Input: part model. Units: mm. Frame: model coordinates. A direction names the side the tool comes from. Round coordinates to 2 decimals unless told otherwise and drop trailing zeros. Loops run counter-clockwise (first coordinate to the right, second up) from the corner with the lowest first, then second, coordinate; pieces in that order, holes last. Notation, with made-up numbers: M -17,8.25 L 8,8.25 A25 cw 8,25.25 Z; hole C -30.5,66.5 d11. An arc over 180 degrees is marked long. Use one line per item in the form item = value. Start each with the question number.
Q1. Access query for faces 1 (the flat face through (24, 1, 0)), 2 (the flat face through (-46, 12.7, 82)), 3 (the flat face through (25, 1, 25.4)). Directions: +Z, -Z, +X, -X, +Y, -Y. A direction counts if a zero-diameter tool reaches every point of the face in a straight line with its end or side. Return the directions, or none.
Q2. Section query B-B, the plane z = 75. Output: boundary loops of the cut face in (x, y), and give its area (3 significant figures).
Q3. Section query A-A, the plane x = -0.5. Output: boundary loops of the cut face in (y, z), and give its area (3 significant figures).
Q4. First-contact query: P1, Ø5, axis at y = 14.5, z = 107.5, coming from the +X side; P2, Ø3, axis at x = -18.5, y = 2, coming from the +Z side; P3, Ø4, axis at x = -41.5, y = -29.5, coming from the +Z side. Flat tips, straight axial feed; report the tip coordinate or a pass-through.
Q5. Section query D-D, the plane y = 19.5. Output: boundary loops of the cut face in (x, z).
Q6. Mould query, pull axis X, two halves, no side actions, for faces 4 (the cylindrical face through (-45.87, -43.16, 119.76)), 5 (the cylindrical face through (6.72, 40.54, 12.88)), 6 (the flat face through (-58.395, 23, 83)), 7 (the flat face through (62.344, 44.361, 12.522)). Classes: pulls with the +X half, pulls with the -X half, needs draft (parallel to the pull), parting line crosses it, or undercut.
Q7. Ray query, line 1 along Y through (x, z) = (50, 7); line 2 along Y through (x, z) = (0, 19); line 3 along Z through (x, y) = (42.5, 4). Return the intervals inside material, ascending.
Q8. Section query C-C, the plane y = -30. Output: boundary loops of the cut face in (x, z).
```python
from build123d import *

# Parameters (mm, degrees)
F1_DEPTH      = 50.8
F1_DEPTH_BACK = 50.8
F3_DEPTH      = 25.4
F4_R          = 12.5
F5_DEPTH      = 25.4
F6_R          = 25.4
F7_SIZE       = 12.7


with BuildPart() as f1:
    # F0 (on Front) → F1 (new body, two sides)
    with BuildSketch(Plane.XZ) as f1_sk:
        with BuildLine():
            Line((-32.9945316374, 127), (-58.3945316374, 127))
            Line((-58.3945316374, 127), (-58.3945316374, 38.1))
            ThreePointArc((-58.3945316374, 38.1), (-47.2353000006, 11.1592316368), (-20.2945316374, 0))
            Line((-20.2945316374, 0), (68.6054683626, 0))
            Line((68.6054683626, 0), (68.6054683626, 25.4))
            Line((68.6054683626, 25.4), (-20.2945316374, 25.4))
            ThreePointArc((-20.2945316374, 25.4), (-29.2747877585, 29.1197438789), (-32.9945316374, 38.1))
            Line((-32.9945316374, 38.1), (-32.9945316374, 127))
        make_face()
    extrude(amount=-F1_DEPTH)
    extrude(f1_sk.sketch, amount=F1_DEPTH_BACK)

    # F2 (on face) → F3 (cut)
    with BuildSketch(Plane.YZ.offset(-32.9945316374)):
        with BuildLine():
            ThreePointArc((12.7, 101.6), (0, 114.3), (-12.7, 101.6))
            Line((-12.7, 101.6), (-12.7, 63.5))
            ThreePointArc((-12.7, 63.5), (0, 50.8), (12.7, 63.5))
            Line((12.7, 63.5), (12.7, 101.6))
        make_face()
    extrude(amount=-F3_DEPTH, mode=Mode.SUBTRACT)

    # F4 (on face) → F5 (cut)
    with BuildSketch(Plane.XY.offset(25.4)):
        with Locations((0, 30)):
            Circle(F4_R)
        with Locations((50, -30)):
            Circle(F4_R)
    extrude(amount=-F5_DEPTH, mode=Mode.SUBTRACT)

    # F6
    f6_edges = [f1.edges().sort_by_distance(p)[0] for p in [
        (-45.694532, -50.8, 127),
        (-45.694532, 50.8, 127),
    ]]
    fillet(f6_edges, radius=F6_R)

    # F7
    f7_edges = [f1.edges().sort_by_distance(p)[0] for p in [
        (68.605468, -50.8, 12.7),
        (68.605468, 50.8, 12.7),
    ]]
    chamfer(f7_edges, length=F7_SIZE)


solid = f1.part
```
Results found:
q1.face_1 = -Z, +X, -X, +Y, -Y
q1.face_2 = +X, -X
q1.face_3 = +Z, +X, +Y, -Y
q2.outline = M -58.39,-50.8 L -32.99,-50.8 L -32.99,-12.7 L -58.39,-12.7 Z; M -58.39,12.7 L -32.99,12.7 L -32.99,50.8 L -58.39,50.8 Z
q2.area = 1,940 mm²
q3.outline = M -50.8,0 L 17.51,0 L 17.51,25.4 L -50.8,25.4 Z; M 42.49,0 L 50.8,0 L 50.8,25.4 L 42.49,25.4 Z
q3.area = 1,950 mm²
q4.P1 = -32.99
q4.P2 = 25.4
q4.P3 = 126.91
q5.outline = M -58.39,38.1 A38.1 ccw -20.29,0 L -6.78,0 L -6.78,25.4 L -20.29,25.4 A12.7 cw -32.99,38.1 L -32.99,127 L -58.39,127 Z; M 6.78,0 L 68.61,0 L 68.61,25.4 L 6.78,25.4 Z
q6.face_4 = needs draft
q6.face_5 = undercut
q6.face_6 = pulls with the -X half
q6.face_7 = pulls with the +X half
q7.line_1 = -50.8 to -42.5, -17.5 to 50.8
q7.line_2 = -50.8 to 17.5, 42.5 to 50.8
q7.line_3 = 0 to 25.4
q8.outline = M -58.39,38.1 A38.1 ccw -20.29,0 L 37.5,0 L 37.5,25.4 L -20.29,25.4 A12.7 cw -32.99,38.1 L -32.99,126.58 L -58.39,126.58 Z; M 62.5,0 L 68.61,0 L 68.61,25.4 L 62.5,25.4 Z
